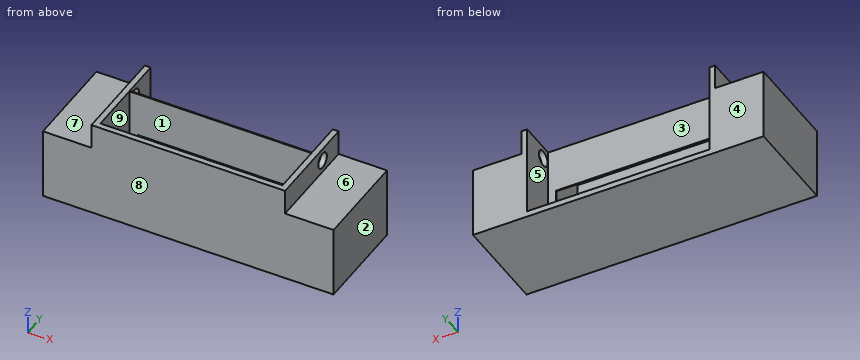
```python
from build123d import *

# Parameters (mm, degrees)
SKETCH1_W           = 100
SKETCH1_H           = 40
BOSS_EXTRUDE1_DEPTH = 50
SKETCH2_W           = 94
SKETCH2_H           = 47
CUT_EXTRUDE1_DEPTH  = 37
SKETCH3_W           = 37
SKETCH3_H           = 40
BOSS_EXTRUDE2_DEPTH = 25
SKETCH4_R           = 4
CUT_EXTRUDE2_DEPTH  = 137.106575888
BOSS_EXTRUDE3_DEPTH = 10
BOSS_EXTRUDE4_REACH = 97
SKETCH7_W           = 94
SKETCH7_H           = 0.5
CUT_EXTRUDE3_REACH  = 97.159
SKETCH8_W           = 85.699881722
SKETCH8_H           = 22.040366035


with BuildPart() as part:
    # Sketch1 → Boss-Extrude1 (new body)
    with BuildSketch(Plane.XY):
        Rectangle(SKETCH1_W, SKETCH1_H)
    extrude(amount=-BOSS_EXTRUDE1_DEPTH)

    # Sketch2 → Cut-Extrude1 (cut)
    with BuildSketch(Plane(origin=(0, 20, 0), x_dir=(1, 0, 0), z_dir=(0, 1, 0))):
        with Locations((0, 23.5)):
            Rectangle(SKETCH2_W, SKETCH2_H)
    extrude(amount=-CUT_EXTRUDE1_DEPTH, mode=Mode.SUBTRACT)

    # Sketch3 → Boss-Extrude2 (add)
    with BuildSketch(Plane(origin=(50, 0, 0), x_dir=(0, 0, -1), z_dir=(1, 0, 0))):
        with Locations((31.5, 0)):
            Rectangle(SKETCH3_W, SKETCH3_H)
    boss_extrude2 = extrude(amount=BOSS_EXTRUDE2_DEPTH)

    # Mirror2: Boss-Extrude2 across plane
    add(boss_extrude2.mirror(Plane.ZY))

    # Sketch4 → Cut-Extrude2 (cut, through all)
    with BuildSketch(Plane.ZY.offset(50)):
        with Locations(Location((-6.5, 15, 0), (0, 0, 90))):
            Circle(SKETCH4_R)
    extrude(amount=-CUT_EXTRUDE2_DEPTH, mode=Mode.SUBTRACT)

    # Sketch6 → Boss-Extrude3 (add)
    with BuildSketch(Plane(origin=(0, 20, 0), x_dir=(1, 0, 0), z_dir=(0, 1, 0))):
        Polygon((-47, 0), (-47, 47), (47, 47), (47, 0), (50, 0), (50, 13), (75, 13), (75, 50), (-75, 50), (-75, 13), (-50, 13), (-50, 0), align=None)
    extrude(amount=BOSS_EXTRUDE3_DEPTH)

    # Sketch7 → Boss-Extrude4 (add, up to next)
    with BuildSketch(Plane.XY, mode=Mode.PRIVATE) as boss_extrude4_sk1:
        with Locations((0, 10.25)):
            Rectangle(SKETCH7_W, SKETCH7_H)
    boss_extrude4_tool1 = extrude(boss_extrude4_sk1.sketch, amount=-BOSS_EXTRUDE4_REACH, mode=Mode.PRIVATE) - part.part
    add(boss_extrude4_tool1.solids().sort_by_distance((0, 10.25, 0))[0])

    # Sketch8 → Cut-Extrude3 (cut, up to next)
    with BuildSketch(Plane(origin=(0, 10.5, 0), x_dir=(1, 0, 0), z_dir=(0, 1, 0)), mode=Mode.PRIVATE) as cut_extrude3_sk1:
        with Locations((0, 34.43157355)):
            Rectangle(SKETCH8_W, SKETCH8_H)
    cut_extrude3_tool1 = extrude(cut_extrude3_sk1.sketch, amount=-CUT_EXTRUDE3_REACH, mode=Mode.PRIVATE) & part.part
    add(cut_extrude3_tool1.solids().sort_by_distance((0, 10.5, -34.431574))[0], mode=Mode.SUBTRACT)


solid = part.part
```
Can you work these out from the model? Positions are in its coordinate system, mm. Face numbers are marked on the shaded views. A direction names the side the tool comes from. Coordinates: 2 decimals unless noted, no trailing zeros. Loops run counter-clockwise (first coordinate to the right, second up) from the corner with the lowest first, then second, coordinate; pieces in that order, holes last. Notation, with made-up numbers: (12, 80.25) -> (56, 80.25) arc R29 cw to (56, 111.25) -> close; hole circle Ø7 at (54, 39.5). An arc over 180 degrees is marked (long way). Answer as a JSON object with one key per item and string values.
1) For the marked faces 5, 6, 7, 8 and 9, which set-ups out of +Z, -Z, +X, -X, +Y, -Y let a thin tool reach every point of the face, with its end or its side?
Results:
{"face 5": "+Z, +Y", "face 6": "+Z, +X, +Y, -Y", "face 7": "+Z, -X, +Y, -Y", "face 8": "+Z, -Z, +X, -X, -Y", "face 9": "+Z"}
2) Imagine slicing it at C-C (y = 15). Please give me the cut outline in (x, z), then the cut area to 3 significant figures.
Results:
{"outline": "(-75, -50) -> (75, -50) -> (75, -13) -> (50, -13) -> (50, -10.5) -> (47, -10.5) -> (47, -47) -> (-47, -47) -> (-47, -10.5) -> (-50, -10.5) -> (-50, -13) -> (-75, -13) -> close; (-50, -2.5) -> (-47, -2.5) -> (-47, 0) -> (-50, 0) -> close; (47, -2.5) -> (50, -2.5) -> (50, 0) -> (47, 0) -> close", "area": "2,380 mm^2"}
3) For P1, Ø4, axis at y = -5.5, z = -7.5, coming from the -X side; P2, Ø12, axis at x = 57, y = 9.5, coming from the +Z side; P3, Ø4, axis at x = 28, y = 18, coming from the +Z side; P4, Ø5, axis at y = 15, z = -6.5, coming from the -X side, each with a flat end and sliding along its axis, tell me the tip position at first contact or that it passes through.
Results:
{"P1": "stops at x = -50", "P2": "stops at z = -13", "P3": "stops at z = -47", "P4": "passes through"}
4) Thinking about a two-plate mould opening in X: for the marked faces 1, 2, 3 and 4, which applies, pulls with the +X half, pulls with the -X half, needs draft (parallel to the pull), parting line crosses it, or undercut?
Results:
{"face 1": "undercut", "face 2": "pulls with the +X half", "face 3": "undercut", "face 4": "needs draft"}
5) Imagine slicing it at A-A (z = -6.5). Please give me the cut outline in (x, y), then the cut area to 3 significant figures.
Results:
{"outline": "(-50, -20) -> (50, -20) -> (50, 11) -> (47, 11) -> (47, 10.5) -> (-47, 10.5) -> (-47, 11) -> (-50, 11) -> close; (-50, 19) -> (-47, 19) -> (-47, 30) -> (-50, 30) -> close; (47, 19) -> (50, 19) -> (50, 30) -> (47, 30) -> close; hole (-47, -17) -> (47, -17) -> (47, 10) -> (-47, 10) -> close", "area": "581 mm^2"}
6) If I drill on line 1 (Z direction, x = 49, y = 15); line 2 (X direction, y = 17, z = -46); line 3 (X direction, y = 24, z = -8), over which ranges is the centre line in solid material (lowest first)?
Results:
{"line 1": "z = -50 to -10.5, -2.5 to 0", "line 2": "x = -75 to -47, 47 to 75", "line 3": "x = -50 to -47, 47 to 50"}
7) Imagine slicing it at D-D (z = -30.5). Please give me the cut outline in (x, y).
Results:
{"outline": "(-75, -20) -> (75, -20) -> (75, 30) -> (47, 30) -> (47, 10.5) -> (42.85, 10.5) -> (42.85, 10) -> (47, 10) -> (47, -17) -> (-47, -17) -> (-47, 10) -> (-42.85, 10) -> (-42.85, 10.5) -> (-47, 10.5) -> (-47, 30) -> (-75, 30) -> close"}
8) Imagine slicing it at B-B (x = -2). Please give me the cut outline in (y, z), then the cut area to 3 significant figures.
Results:
{"outline": "(-20, -50) -> (30, -50) -> (30, -47) -> (10.5, -47) -> (10.5, -45.45) -> (10, -45.45) -> (10, -47) -> (-17, -47) -> (-17, 0) -> (-20, 0) -> close; (10, -23.41) -> (10.5, -23.41) -> (10.5, 0) -> (10, 0) -> close", "area": "303 mm^2"}
